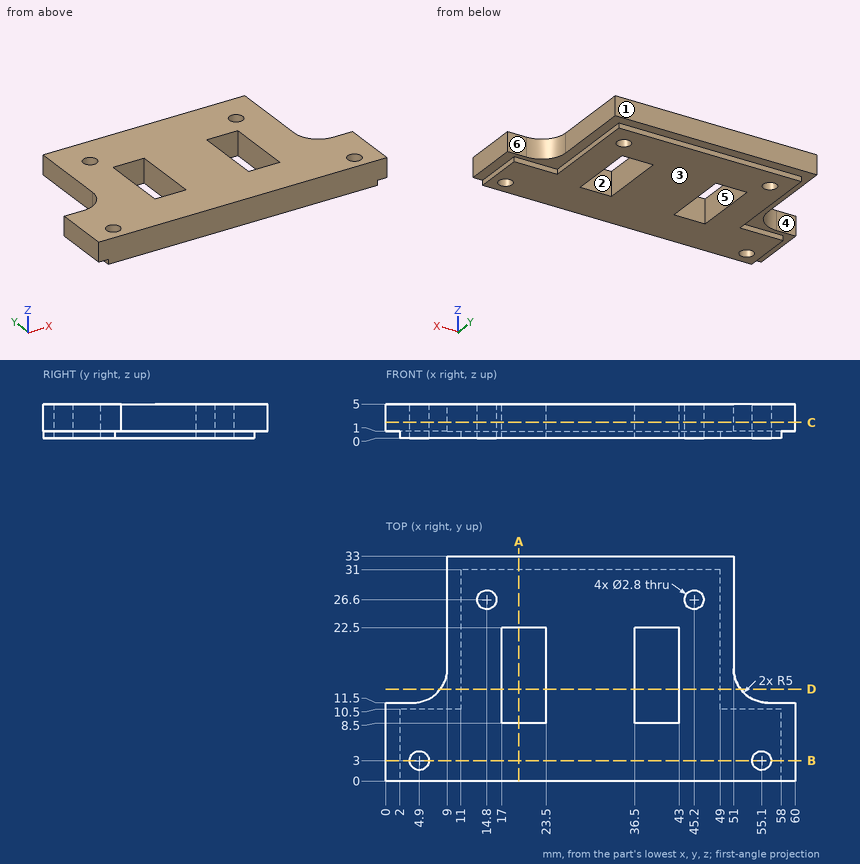
Could you check a few things on this drawing? It's one solid part, dimensions in mm from its lowest x, y, z. A direction names the side the tool comes from. Coordinates: 2 decimals unless noted, no trailing zeros. Order: outer loops, then holes, each group sorted by start corner. A loop starts at its lowest first (then second) coordinate and runs counter-clockwise, first axis right, second up. Notation, with made-up numbers: (-9, -14) -> (10, -14) arc R17 cw to (10, 12) -> close; hole circle Ø7 at (49, 1.25). An arc over 180 degrees is marked (long way). One line per item, written item: value. Start each with the question number.
1) Imagine slicing it at B-B on y = 3. List the corners of the cut face in (x, z) for me.
2) If I drill on L1, parallel to X at y = 18, z = 0.2; L2, parallel to Y at x = 19, z = 3.25; L3, parallel to X at y = 3.5, z = 3.4, over which ranges is the centre line in solid material (lowest first)? Write a range as [from, to].
3) I'm going to push flat-ended pins straight in: pin 1 (0.8 mm diameter, centred on y = 20, z = 0.5, fed in from +X); pin 2 (0.8 mm diameter, centred on x = 55.5, z = 0.5, fed in from +Y); pin 3 (1.2 mm diameter, centred on y = 23, z = 4, fed in from +X); pin 4 (2 mm diameter, centred on x = 45.2, y = 26.6, fed in from +Z). Where does each tip first touch, or does it pass through?
4) Imagine slicing it at C-C on z = 2.3. List the corners of the cut face in (x, y) for me.
5) Imagine slicing it at D-D on y = 13.5. List the corners of the cut face in (x, z) for me, plus the area to 3 significant figures.
6) We'd pull the mould along Y, two halves only. Please class the marked faces 1, 2 and 3: +Y half, -Y half, draft (parallel to the pull), parting line (faces both ways), or undercut.
7) Which directions (+Z, -Z, +X, -X, +Y, -Y) give clear straight access to the entire face, cutting with the end or side of a thin tool? Please do the marked faces 4, 5 and 6.
8) Imagine slicing it at A-A on x = 19.5. List the corners of the cut face in (y, z) for me.
Answer list:
1. outline: (0, 1) -> (2, 1) -> (2, 0) -> (3.5, 0) -> (3.5, 5) -> (0, 5) -> close; (6.3, 0) -> (53.7, 0) -> (53.7, 5) -> (6.3, 5) -> close; (56.5, 0) -> (58, 0) -> (58, 1) -> (60, 1) -> (60, 5) -> (56.5, 5) -> close
2. L1: x = [11, 17], [23.5, 36.5], [43, 49]
2. L2: y = [0, 8.5], [22.5, 33]
2. L3: x = [0, 3.59], [6.21, 53.79], [56.41, 60]
3. pin 1: stops at x = 49
3. pin 2: stops at y = 10.5
3. pin 3: stops at x = 51
3. pin 4: passes through
4. outline: (0, 0) -> (60, 0) -> (60, 11.5) -> (56, 11.5) arc R5 cw to (51, 16.5) -> (51, 33) -> (9, 33) -> (9, 16.5) arc R5 cw to (4, 11.5) -> (0, 11.5) -> close; hole circle Ø2.8 at (4.9, 3); hole circle Ø2.8 at (14.8, 26.6); hole (17, 8.5) -> (23.5, 8.5) -> (23.5, 22.5) -> (17, 22.5) -> close; hole (36.5, 8.5) -> (43, 8.5) -> (43, 22.5) -> (36.5, 22.5) -> close; hole circle Ø2.8 at (45.2, 26.6); hole circle Ø2.8 at (55.1, 3)
5. outline: (8, 1) -> (11, 1) -> (11, 0) -> (17, 0) -> (17, 5) -> (8, 5) -> close; (23.5, 0) -> (36.5, 0) -> (36.5, 5) -> (23.5, 5) -> close; (43, 0) -> (49, 0) -> (49, 1) -> (52, 1) -> (52, 5) -> (43, 5) -> close
5. area: 149 mm2
6. face 1: +Y half
6. face 2: undercut
6. face 3: draft
7. face 4: +Z, -Z, -X, +Y
7. face 5: +Z, -Z
7. face 6: +Z, -Z, +X, +Y
8. outline: (0, 0) -> (8.5, 0) -> (8.5, 5) -> (0, 5) -> close; (22.5, 0) -> (31, 0) -> (31, 1) -> (33, 1) -> (33, 5) -> (22.5, 5) -> close
